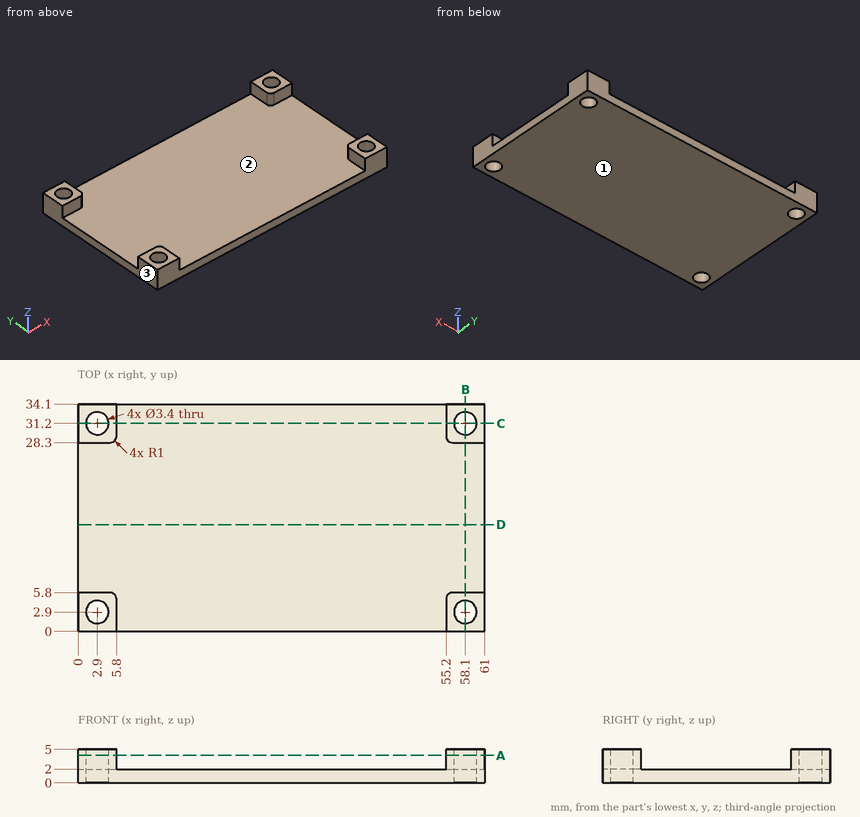
Job drawing, mm, ordinate dimensions from the low corner. One solid piece. Coordinates: 2 decimals unless noted, no trailing zeros. Write each loop counter-clockwise with the first axis right and the second up, starting at its lowest first coordinate (ties: lowest second). Pieces come first, ordered by that corner, then holes. Notation, with made-up numbers: (22.5, 75.5) - (54.5, 75.5) arc R32 ccw to (54.5, 106.5) - close; hole circle Ø7 at (69.25, 41.5). An arc over 180 degrees is marked (long way). Use a Markdown table: item, result. Add a question column.
Item 1: Flat gauge pins, fed straight in: pin 1 (3 mm diameter, centred on x = 58.1, y = 31.2, fed in from +Z); pin 2 (6 mm diameter, centred on x = 6, y = 13, fed in from +Z). Where does each tip first touch, or does it go through?
Item 2: Band-saw the part on B-B, the plane x = 58.1. Give the cut face in (y, z), and give its area (3 significant figures).
Item 3: Drill centre lines: L1, parallel to Y at x = 2.9, z = 3.75; L2, parallel to Y at x = 2.9, z = 1.5; L3, parallel to Y at x = 3.5, z = 3.4. Where is each one in solid material? Low to high. Write a range as from..to.
Item 4: Band-saw the part on C-C, the plane y = 31.2. Give the cut face in (x, z).
Item 5: Band-saw the part on D-D, the plane y = 16. Give the cut face in (x, z), and give its area (3 significant figures).
Item 6: Band-saw the part on A-A, the plane z = 4.1. Give the cut face in (x, y), and give its area (3 significant figures).
Item 7: Mould opens along X. For the marked faces 1, 2 and 3 say: pulls with the +X half, pulls with the -X half, needs draft (parallel to the pull), parting line crosses it, or undercut.
Numbers:
| question | item | result |
|---|---|---|
| 1 | pin 1 | through |
| 1 | pin 2 | z = 2 |
| 2 | outline | (0, 0) - (1.2, 0) - (1.2, 5) - (0, 5) - close; (4.6, 0) - (29.5, 0) - (29.5, 5) - (28.3, 5) - (28.3, 2) - (5.8, 2) - (5.8, 5) - (4.6, 5) - close; (32.9, 0) - (34.1, 0) - (34.1, 5) - (32.9, 5) - close |
| 2 | area | 69.0 mm2 |
| 3 | L1 | 0..1.2, 4.6..5.8, 28.3..29.5, 32.9..34.1 |
| 3 | L2 | 0..1.2, 4.6..29.5, 32.9..34.1 |
| 3 | L3 | 0..1.31, 4.49..5.8, 28.3..29.61, 32.79..34.1 |
| 4 | outline | (0, 0) - (1.2, 0) - (1.2, 5) - (0, 5) - close; (4.6, 0) - (56.4, 0) - (56.4, 5) - (55.2, 5) - (55.2, 2) - (5.8, 2) - (5.8, 5) - (4.6, 5) - close; (59.8, 0) - (61, 0) - (61, 5) - (59.8, 5) - close |
| 5 | outline | (0, 0) - (61, 0) - (61, 2) - (0, 2) - close |
| 5 | area | 122 mm2 |
| 6 | outline | (0, 0) - (5.8, 0) - (5.8, 4.8) arc R1 ccw to (4.8, 5.8) - (0, 5.8) - close; (0, 28.3) - (4.8, 28.3) arc R1 ccw to (5.8, 29.3) - (5.8, 34.1) - (0, 34.1) - close; (55.2, 0) - (61, 0) - (61, 5.8) - (56.2, 5.8) arc R1 ccw to (55.2, 4.8) - close; (55.2, 29.3) arc R1 ccw to (56.2, 28.3) - (61, 28.3) - (61, 34.1) - (55.2, 34.1) - close; hole circle Ø3.4 at (2.9, 2.9); hole circle Ø3.4 at (2.9, 31.2); hole circle Ø3.4 at (58.1, 2.9); hole circle Ø3.4 at (58.1, 31.2) |
| 6 | area | 97.4 mm2 |
| 7 | face 1 | needs draft |
| 7 | face 2 | undercut |
| 7 | face 3 | pulls with the -X half |
